Input: dimensioned drawing with shaded views. Units: mm. Origin: part minimum x, y, z. A direction names the side the tool comes from. Round coordinates to 2 decimals unless told otherwise and drop trailing zeros. Loops run counter-clockwise (first coordinate to the right, second up) from the corner with the lowest first, then second, coordinate; pieces in that order, holes last. Notation, with made-up numbers: (-17, -15) - (26, -15) arc R19 cw to (26, 15) - close; hole circle Ø3 at (76, -3.75). An arc over 180 degrees is marked (long way). One line per question, with ' | ' between items. Start each with the question number.
1. Cut plane A-A (x = 37). Return loops of the section in (y, z).
2. Access query for the marked faces 1 and 2. Directions: +Z, -Z, +X, -X, +Y, -Y. A direction counts if a zero-diameter tool reaches every point of the face in a straight line with its end or side. Return the directions, or none.
3. Ray query, line 1 (X direction, y = 4, z = 49); line 2 (Y direction, x = 197, z = 4); line 3 (Y direction, x = 24.5, z = 17). Return the intervals inside material, ascending.
4. Cut plane B-B (y = 80). Return loops of the section in (x, z).
5. Cut plane D-D (y = 19). Return loops of the section in (x, z), then the cut area to 3 significant figures.
6. Pin query (flat end, axial travel): pin 1 (2 mm diameter, centred on x = 153, y = 43.5, fed in from +Z); pin 2 (21 mm diameter, centred on x = 37, z = 49, fed in from +Y); pin 3 (6 mm diameter, centred on x = 95, z = 52, fed in from +Y). Return the tip coordinate at first contact, or that it passes through.
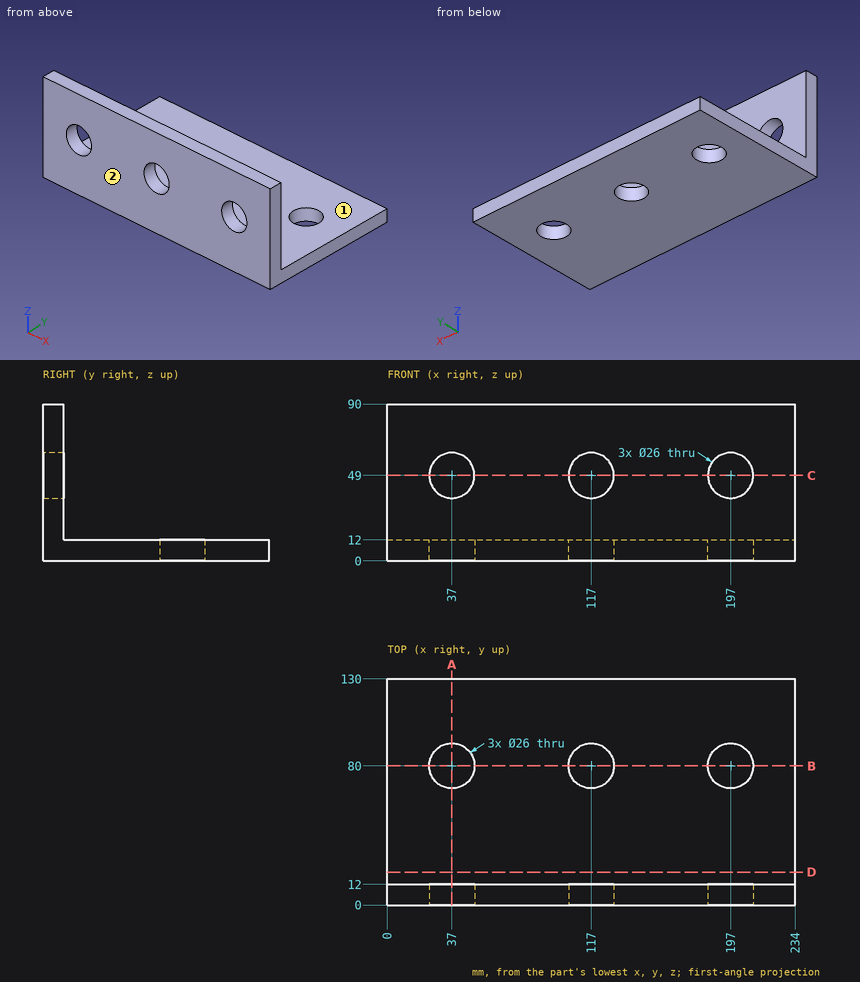
Answers follow:
1) outline: (0, 0) - (67, 0) - (67, 12) - (12, 12) - (12, 36) - (0, 36) - close; (0, 62) - (12, 62) - (12, 90) - (0, 90) - close; (93, 0) - (130, 0) - (130, 12) - (93, 12) - close
2) face 1: +Z, +X, -X, +Y | face 2: +Z, -Z, +X, -X, -Y
3) line 1: x = 0 to 24, 50 to 104, 130 to 184, 210 to 234 | line 2: y = 0 to 67, 93 to 130 | line 3: y = 0 to 12
4) outline: (0, 0) - (24, 0) - (24, 12) - (0, 12) - close; (50, 0) - (104, 0) - (104, 12) - (50, 12) - close; (130, 0) - (184, 0) - (184, 12) - (130, 12) - close; (210, 0) - (234, 0) - (234, 12) - (210, 12) - close
5) outline: (0, 0) - (234, 0) - (234, 12) - (0, 12) - close | area: 2,810 mm2
6) pin 1: stops at z = 12 | pin 2: passes through | pin 3: stops at y = 12
